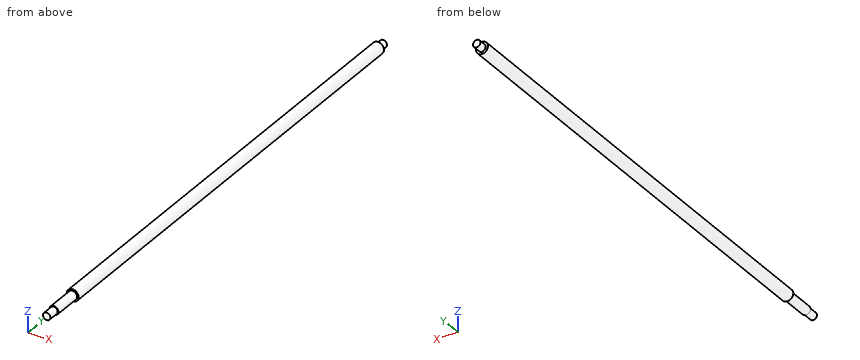
```python
from build123d import *

# Parameters (mm, degrees)
SKETCH_R     = 5
PAD_DEPTH    = 15
SKETCH001_R  = 6
PAD001_DEPTH = 39
SKETCH002_R  = 8
PAD002_DEPTH = 635
SKETCH003_R  = 5
PAD003_DEPTH = 11


with BuildPart() as part:
    # Sketch → Pad (new body)
    with BuildSketch(Plane.XZ):
        Circle(SKETCH_R)
    extrude(amount=-PAD_DEPTH)

    # Sketch001 (on Face3 of Pad) → Pad001 (join)
    with BuildSketch(Plane(origin=(0, 15, 0), x_dir=(1, 0, 0), z_dir=(0, 1, 0))):
        Circle(SKETCH001_R)
    extrude(amount=PAD001_DEPTH)

    # Sketch002 (on Face3 of Pad001) → Pad002 (join)
    with BuildSketch(Plane(origin=(0, 54, 0), x_dir=(1, 0, 0), z_dir=(0, 1, 0))):
        Circle(SKETCH002_R)
    extrude(amount=PAD002_DEPTH)

    # Sketch003 (on Face3 of Pad002) → Pad003 (join)
    with BuildSketch(Plane(origin=(0, 689, 0), x_dir=(1, 0, 0), z_dir=(0, 1, 0))):
        Circle(SKETCH003_R)
    extrude(amount=PAD003_DEPTH)


solid = part.part
```
The listing builds one solid part. Answer for the finished solid, in the listing's coordinates (mm). Give positions to 0.01 mm unless a question says otherwise; leave off trailing zeros. Order: outer loops, then holes, each group sorted by start corner. A loop starts at its lowest first (then second) coordinate and runs counter-clockwise, first axis right, second up. Notation, with made-up numbers: (5, -9.75) -> (21, -9.75) arc R19 cw to (21, 9.25) -> close; hole circle Ø8 at (-11.75, 71.25). An arc over 180 degrees is marked (long way). One line per item, written item: value.
1) Find the intervals of material crossed by line 1 (X direction, y = 316.5, z = 1); line 2 (Y direction, x = 2, z = 6.75); line 3 (X direction, y = 518, z = -0.5), in increasing order.
Reported:
line 1: x = -7.94 to 7.94
line 2: y = 54 to 689
line 3: x = -7.98 to 7.98
2) Find section A-A, the plane x = 0. Determine the outline of the cut face in (y, z).
Reported:
outline: (0, -5) -> (15, -5) -> (15, -6) -> (54, -6) -> (54, -8) -> (689, -8) -> (689, -5) -> (700, -5) -> (700, 5) -> (689, 5) -> (689, 8) -> (54, 8) -> (54, 6) -> (15, 6) -> (15, 5) -> (0, 5) -> close
3) Flat-ended cylindrical pins translate along their axes: P1, Ø2, axis at x = 5, y = 540.5, coming from the +Z side; P2, Ø4, axis at y = 137, z = -5.5, coming from the -X side; P3, Ø3, axis at x = 5, y = 359, coming from the +Z side. Find the tip coordinate at first contact, or state that the pin passes through.
Reported:
P1: stops at z = 6.93
P2: stops at x = -7.19
P3: stops at z = 7.19
4) Find section C-C, the plane y = 586. Determine the outline of the cut face in (x, z).
Reported:
outline: circle Ø16 at (0, 0)
5) Find section B-B, the plane z = 0. Determine the outline of the cut face in (x, y).
Reported:
outline: (-8, 54) -> (-6, 54) -> (-6, 15) -> (-5, 15) -> (-5, 0) -> (5, 0) -> (5, 15) -> (6, 15) -> (6, 54) -> (8, 54) -> (8, 689) -> (5, 689) -> (5, 700) -> (-5, 700) -> (-5, 689) -> (-8, 689) -> close
